from build123d import *

# Parameters (mm, degrees)
SKETCH3_W               = 90
SKETCH3_H               = 52
BOSS_EXTRUDE2_DEPTH     = 2
FILLET2_R               = 2
BOSS_EXTRUDE3_START     = 2
SKETCH7_R               = 4
BOSS_EXTRUDE3_DEPTH     = 10
CUT_EXTRUDE2_DEPTH      = 54.338541412
CUT_EXTRUDE2_DEPTH_BACK = 4
CUT_EXTRUDE2_START      = 2
SKETCH8_R               = 2.35
BOSS_EXTRUDE4_START     = 2
SKETCH10_W              = 83.8
SKETCH10_H              = 45.8
SKETCH10_W_2            = 81
SKETCH10_H_2            = 43
BOSS_EXTRUDE4_DEPTH     = 1
BOSS_EXTRUDE5_START     = 2
SKETCH11_R              = 2.5
BOSS_EXTRUDE5_DEPTH     = 10
CUT_EXTRUDE3_START      = 12
SKETCH12_R              = 1.075
CUT_EXTRUDE3_DEPTH      = 10
SKETCH4_W               = 83
SKETCH4_H               = 45
CUT_EXTRUDE4_DEPTH      = 0.5
CUT_EXTRUDE5_DEPTH      = 54.338541412
CUT_EXTRUDE5_DEPTH_BACK = 54.338541412
SKETCH5_R               = 8
SKETCH5_W               = 18.5
SKETCH5_H               = 18.5


with BuildPart() as part:
    # Sketch3 → Boss-Extrude2 (new body)
    with BuildSketch(Plane(origin=(0, 0, 0), x_dir=(1, 0, 0), z_dir=(0, 1, 0))):
        Rectangle(SKETCH3_W, SKETCH3_H)
    extrude(amount=BOSS_EXTRUDE2_DEPTH)

    # Fillet2
    fillet2_edges = [part.edges().sort_by_distance(p)[0] for p in [
        (-45, 1, -26),
        (45, 1, -26),
        (45, 1, 26),
        (-45, 1, 26),
    ]]
    fillet(fillet2_edges, radius=FILLET2_R)

    # Sketch7 → Boss-Extrude3 (add)
    with BuildSketch(Plane(origin=(0, 0, 0), x_dir=(1, 0, 0), z_dir=(0, 1, 0)).offset(BOSS_EXTRUDE3_START)):
        with Locations(Location((37, 18, 0), (0, 0, 270))):
            Circle(SKETCH7_R)
        with Locations(Location((37, -16.5, 0), (0, 0, 270))):
            Circle(SKETCH7_R)
    extrude(amount=BOSS_EXTRUDE3_DEPTH)

    # Sketch8 → Cut-Extrude2 (cut, two sides: drawn at the far end of the back side and taken through both)
    with BuildSketch(Plane(origin=(0, 0, 0), x_dir=(1, 0, 0), z_dir=(0, 1, 0)).offset(CUT_EXTRUDE2_START - CUT_EXTRUDE2_DEPTH_BACK)):
        with Locations(Location((37, 18, 0), (0, 0, 270))):
            Circle(SKETCH8_R)
        with Locations(Location((37, -16.5, 0), (0, 0, 270))):
            Circle(SKETCH8_R)
    extrude(amount=CUT_EXTRUDE2_DEPTH + CUT_EXTRUDE2_DEPTH_BACK, mode=Mode.SUBTRACT)

    # Sketch10 → Boss-Extrude4 (add)
    with BuildSketch(Plane(origin=(0, 0, 0), x_dir=(1, 0, 0), z_dir=(0, 1, 0)).offset(BOSS_EXTRUDE4_START)):
        Rectangle(SKETCH10_W, SKETCH10_H)
        Rectangle(SKETCH10_W_2, SKETCH10_H_2, mode=Mode.SUBTRACT)
    extrude(amount=BOSS_EXTRUDE4_DEPTH)

    # Sketch11 → Boss-Extrude5 (add)
    with BuildSketch(Plane(origin=(0, 0, 0), x_dir=(1, 0, 0), z_dir=(0, 1, 0)).offset(BOSS_EXTRUDE5_START)):
        with Locations(Location((-29, -19.5, 0), (0, 0, 233.130102354))):
            Circle(SKETCH11_R)
    extrude(amount=BOSS_EXTRUDE5_DEPTH)

    # Sketch12 → Cut-Extrude3 (cut)
    with BuildSketch(Plane(origin=(0, 0, 0), x_dir=(1, 0, 0), z_dir=(0, 1, 0)).offset(CUT_EXTRUDE3_START)):
        with Locations(Location((-29, -19.5, 0), (0, 0, 270))):
            Circle(SKETCH12_R)
    extrude(amount=-CUT_EXTRUDE3_DEPTH, mode=Mode.SUBTRACT)

    # Sketch4 → Cut-Extrude4 (cut)
    with BuildSketch(Plane(origin=(0, 0, 0), x_dir=(1, 0, 0), z_dir=(0, 1, 0))):
        Rectangle(SKETCH4_W, SKETCH4_H)
    extrude(amount=CUT_EXTRUDE4_DEPTH, mode=Mode.SUBTRACT)

    # Sketch5 → Cut-Extrude5 (cut, two sides: drawn at the far end of the back side and taken through both)
    with BuildSketch(Plane(origin=(0, 0, 0), x_dir=(1, 0, 0), z_dir=(0, 1, 0)).offset(-CUT_EXTRUDE5_DEPTH_BACK)):
        with Locations(Location((-32.5, -7.5, 0), (0, 0, 180))):
            Circle(SKETCH5_R)
        with Locations((-14.75, 10.5)):
            Rectangle(SKETCH5_W, SKETCH5_H)
        with Locations((23.25, 10.5)):
            Rectangle(SKETCH5_W, SKETCH5_H)
        with Locations((-14.75, -8.5)):
            Rectangle(SKETCH5_W, SKETCH5_H)
        with Locations((23.25, -8.5)):
            Rectangle(SKETCH5_W, SKETCH5_H)
        with Locations((4.25, 10.5)):
            Rectangle(SKETCH5_W, SKETCH5_H)
        with Locations((4.25, -8.5)):
            Rectangle(SKETCH5_W, SKETCH5_H)
    extrude(amount=CUT_EXTRUDE5_DEPTH + CUT_EXTRUDE5_DEPTH_BACK, mode=Mode.SUBTRACT)


solid = part.part
Read the model definition and answer for the solid it produces. Units are mm, in the model's axes. A direction names the side the tool comes from. Round coordinates to 2 decimals unless told otherwise and drop trailing zeros. Write each loop counter-clockwise with the first axis right and the second up, starting at its lowest first coordinate (ties: lowest second). Pieces come first, ordered by that corner, then holes.
1. The part is cut by section A-A, the plane y = 10.75. Determine the outline of the cut face in (x, z) (3 decimals), then the cut area to 3 significant figures.
2. Straight lines are drawn through the part: L1, parallel to Z at x = -20, y = 1; L2, parallel to X at y = 4.75, z = 16.5; L3, parallel to X at y = 2.25, z = 6. For each, find the intervals that lie inside material, in ascending order.
3. Which of the six approach directions +Z, -Z, +X, -X, +Y, -Y give full straight-line access (tool end or side, diameter ignored) to faces 1 (the face through (-1, 0.5, -20)), 2 (the face through (-28.677, 7.07, 20.525)), 3 (the face through (35, 12, -16))?
4. The part is cut by section D-D, the plane x = 9.5. Determine the outline of the cut face in (y, z).
5. Given pin 1 Ø0.8 at (x, y) = (7.5, 2.5) entering from +Z; pin 2 Ø1.5 at (x, z) = (32, -20) entering from +Y, each flat-ended and moving along its own axis, determine where each tip first touches the part or whether it passes through.
6. Determine the mould class of faces 4 (the face through (44.4, 1.01, 25.43)), 5 (the face through (-29, 7, 17)), 6 (the face through (-44.43, 1.01, -25.4)), 7 (the face through (-26.151, 1.239, 2.632)) for opening direction X: pulls with the +X half, pulls with the -X half, needs draft (parallel to the pull), parting line crosses it, or undercut.
7. The part is cut by section C-C, the plane x = -32.5. Determine the outline of the cut face in (y, z).
8. The part is cut by section B-B, the plane z = -18. State how many separate pieces and enclosed holes the cut face has, then the cut area to 3 significant figures.
Values:
1. outline: circle Ø5 at (-29, 19.5); circle Ø8 at (37, -18); circle Ø8 at (37, 16.5); hole circle Ø2.15 at (-29, 19.5); hole circle Ø4.7 at (37, -18); hole circle Ø4.7 at (37, 16.5)
1. area: 81.8 mm2
2. L1: z = -26 to -19.75, -1.25 to -0.75, 17.75 to 26
2. L2: x = 33 to 34.65, 39.35 to 41
2. L3: x = -41.9 to -40.5, 40.5 to 41.9
3. face 1: -Y
3. face 2: +Y
3. face 3: +Z, -Z, +X, -X, +Y
4. outline: (0, -26) - (2, -26) - (2, -22.9) - (3, -22.9) - (3, -21.5) - (2, -21.5) - (2, -19.75) - (0.5, -19.75) - (0.5, -22.5) - (0, -22.5) - close; (0, 22.5) - (0.5, 22.5) - (0.5, 17.75) - (2, 17.75) - (2, 21.5) - (3, 21.5) - (3, 22.9) - (2, 22.9) - (2, 26) - (0, 26) - close; (0.5, -1.25) - (2, -1.25) - (2, -0.75) - (0.5, -0.75) - close
5. pin 1: stops at z = 22.9
5. pin 2: stops at y = 2
6. face 4: pulls with the +X half
6. face 5: undercut
6. face 6: pulls with the -X half
6. face 7: undercut
7. outline: (0, -26) - (2, -26) - (2, -22.9) - (3, -22.9) - (3, -21.5) - (2, -21.5) - (2, -0.5) - (0.5, -0.5) - (0.5, -22.5) - (0, -22.5) - close; (0, 22.5) - (0.5, 22.5) - (0.5, 15.5) - (2, 15.5) - (2, 21.5) - (3, 21.5) - (3, 22.9) - (2, 22.9) - (2, 26) - (0, 26) - close
8. separate pieces: 5
8. enclosed holes: 0
8. area: 83.5 mm2
